from build123d import *

# Parameters (mm, degrees)
CHANFREIN1_SIZE         = 0.5
ENL_V_MAT_EXTRU_1_DEPTH = 1.8


with BuildPart() as part:
    # Esquisse1 → Révolution1 (revolve)
    with BuildSketch(Plane.XY):
        Polygon((0, 0), (0, 4), (0.3, 4), (2.3, 2), (8, 2), (8, 0), align=None)
    revolve(axis=Axis((8, 0, 0), (-1, 0, 0)))

    # Chanfrein1
    chanfrein1_edges = [part.edges().sort_by_distance(p)[0] for p in [
        (8, -2, 0),
    ]]
    chamfer(chanfrein1_edges, length=CHANFREIN1_SIZE)

    # Esquisse2 → Enlèv. mat.-Extru.1 (cut)
    with BuildSketch(Plane.ZY):
        Polygon((0, 1.443375673), (-1.25, 0.721687836), (-1.25, -0.721687836), (0, -1.443375673), (1.25, -0.721687836), (1.25, 0.721687836), align=None)
    extrude(amount=-ENL_V_MAT_EXTRU_1_DEPTH, mode=Mode.SUBTRACT)


solid = part.part
Can you work these out from the model? Positions are in its coordinate system, mm. A direction names the side the tool comes from. Give positions to 0.01 mm unless a question says otherwise; leave off trailing zeros. Write each loop counter-clockwise with the first axis right and the second up, starting at its lowest first coordinate (ties: lowest second). Pieces come first, ordered by that corner, then holes. Notation, with made-up numbers: (14, -30.75) -> (59, -30.75) arc R22 cw to (59, -24.75) -> close; hole circle Ø11 at (40.5, -15.75). An arc over 180 degrees is marked (long way). Answer as a JSON object with one key per item and string values. Group by question number.
Item 1: Please list where these lines run through material, in increasing order: line 1 (X direction, y = 0, z = -0.75); line 2 (Y direction, x = 1.75, z = -0.25); line 3 (X direction, y = 1.5, z = 2). Write a range as [from, to].
Item 2: We'd pull the mould along Y, two halves only. Please class faces 1 (the face through (0.887, -1.088, 0.616)), 2 (the face through (0.89, -1.08, -0.63)), 3 (the face through (0, -2, 0)), 4 (the face through (5, 0, 2)): +Y half, -Y half, draft (parallel to the pull), parting line (faces both ways), or undercut.
Item 3: Suppose I cut it at A-A (y = 0). Please give me the cut outline in (x, z), plus the area to 4 significant figures.
Item 4: I'm going to push flat-ended pins straight in: P1, Ø2, axis at x = 7, y = 1.5, coming from the +Z side; P2, Ø1.6, axis at x = 0.5, y = 0, coming from the +Z side. Where does each tip first touch, or does it pass through?
Item 5: For faces 5 (the face through (8, 0, 0)), 6 (the face through (1, 0, -1.25)), which set-ups out of +Z, -Z, +X, -X, +Y, -Y let a thin tool reach every point of the face, with its end or its side?
Item 6: Suppose I cut it at B-B (x = 5.5). Please give me the cut outline in (y, z), plus the area to 3 significant figures.
Findings:
{
 "1": {"line 1": "x = [1.8, 8]", "line 2": "y = [-2.54, -1.3], [1.3, 2.54]", "line 3": "x = [0, 1.8]"},
 "2": {"face 1": "undercut", "face 2": "undercut", "face 3": "draft", "face 4": "parting line"},
 "3": {"outline": "(0, -4) -> (0.3, -4) -> (2.3, -2) -> (7.5, -2) -> (8, -1.5) -> (8, 1.5) -> (7.5, 2) -> (2.3, 2) -> (0.3, 4) -> (0, 4) -> (0, 1.25) -> (1.8, 1.25) -> (1.8, -1.25) -> (0, -1.25) -> close", "area": "32.45 mm²"},
 "4": {"P1": "stops at z = 1.94", "P2": "stops at z = 4"},
 "5": {"face 5": "+Z, -Z, +X, +Y, -Y", "face 6": "-X"},
 "6": {"outline": "circle Ø4 at (0, 0)", "area": "12.6 mm²"}
}
